Geometry: see drawing. Coordinates: mm, zero at the bounding-box minimum. Give positions to 0.01 mm unless a question says otherwise; leave off trailing zeros. Loops run counter-clockwise (first coordinate to the right, second up) from the corner with the lowest first, then second, coordinate; pieces in that order, holes last. Notation, with made-up numbers: M 71,77.25 L 86,77.25 A18 ccw 86,93.25 Z; hole C 57.25,51 d11. An arc over 180 degrees is marked long. Answer in a Markdown table with one row per item.
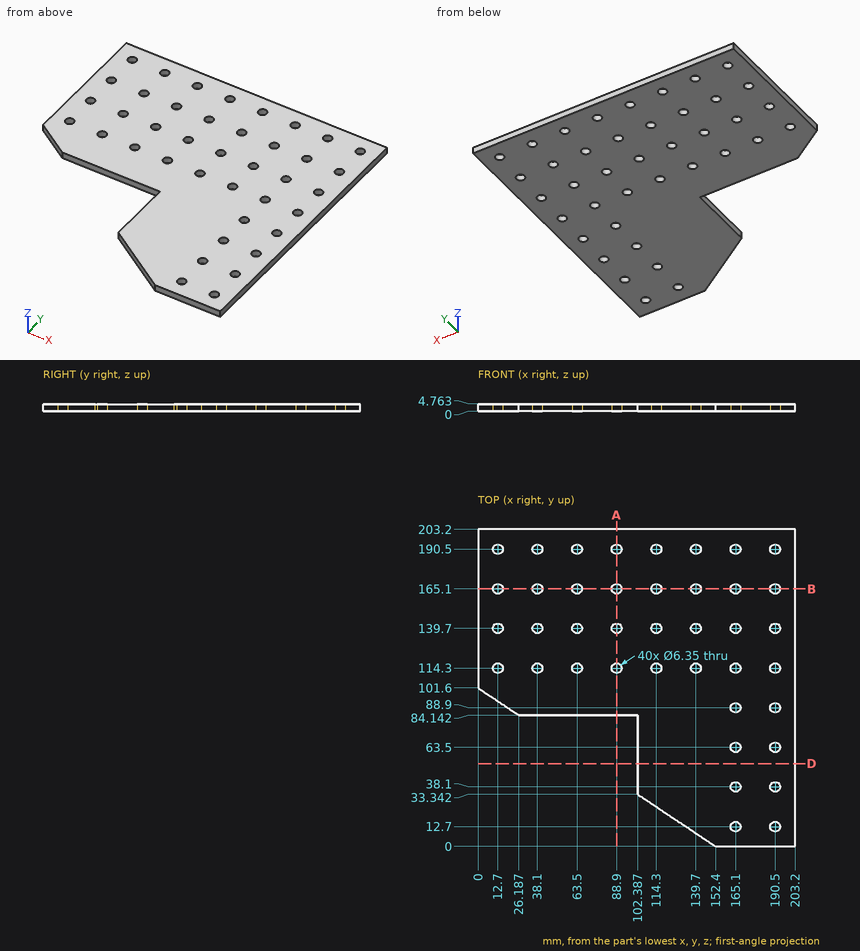
1) Section B-B, the plane y = 165.1. Count the separate pieces of the cut face and the enclosed holes in it.
Reply:
| item | result |
|---|---|
| separate pieces | 9 |
| enclosed holes | 0 |
2) Section A-A, the plane x = 88.9. Return loops of the section in (y, z) (1 decimal), then the cut area to 3 significant figures.
Reply:
| item | result |
|---|---|
| outline | M 84.1,0 L 111.1,0 L 111.1,4.8 L 84.1,4.8 Z; M 117.5,0 L 136.5,0 L 136.5,4.8 L 117.5,4.8 Z; M 142.9,0 L 161.9,0 L 161.9,4.8 L 142.9,4.8 Z; M 168.3,0 L 187.3,0 L 187.3,4.8 L 168.3,4.8 Z; M 193.7,0 L 203.2,0 L 203.2,4.8 L 193.7,4.8 Z |
| area | 446 mm² |
3) Section D-D, the plane y = 53. Return loops of the section in (x, z), then the cut area to 3 significant figures.
Reply:
| item | result |
|---|---|
| outline | M 102.39,0 L 203.2,0 L 203.2,4.76 L 102.39,4.76 Z |
| area | 480 mm² |
4) Material intervals for L1, parallel to X at y = 38.1, z = 1 (1 decimal); L2, parallel to Y at x = 40, z = 1.25 (1 decimal); L3, parallel to X at y = 12, z = 4.5 (1 decimal), sorted ascending.
Reply:
| item | result |
|---|---|
| L1 | x = 102.4 to 161.9, 168.3 to 187.3, 193.7 to 203.2 |
| L2 | y = 84.1 to 111.8, 116.8 to 137.2, 142.2 to 162.6, 167.6 to 188, 193 to 203.2 |
| L3 | x = 134.4 to 162, 168.2 to 187.4, 193.6 to 203.2 |
5) Pin query (flat end, axial travel): pin 1 Ø8.5 at (x, y) = (165.1, 12.7) entering from -Z; pin 2 Ø5 at (x, y) = (190.5, 165.1) entering from +Z; pin 3 Ø2.5 at (x, z) = (74, 2.5) entering from -Y. Return the tip coordinate at first contact, or that it passes through.
Reply:
| item | result |
|---|---|
| pin 1 | stops at z = 0 |
| pin 2 | passes through |
| pin 3 | stops at y = 84.14 |
